from build123d import *

# Parameters (mm, degrees)
ESQUISSE1_R             = 4.25
BOSS_EXTRU_1_DEPTH      = 8
ESQUISSE2_W             = 5.5
ESQUISSE2_H             = 31
BOSS_EXTRU_2_DEPTH      = 1
CHANFREIN1_SIZE         = 1
ESQUISSE3_R             = 2.1
ENL_V_MAT_EXTRU_1_DEPTH = 39.288379438
ENL_V_START             = -5
ESQUISSE4_R             = 4
ENL_V_MAT_EXTRU_2_DEPTH = 33.749172176
CONG_1_R                = 2.5


with BuildPart() as part:
    # Esquisse1 → Boss.-Extru.1 (new, symmetric)
    with BuildSketch(Plane(origin=(0, 0, 0), x_dir=(0, 0, -1), z_dir=(1, 0, 0))):
        with BuildLine():
            Line((0, 0), (0, 31))
            Line((0, 31), (-10, 31))
            ThreePointArc((-10, 31), (-18.331958567, 26.529779962), (-19.214779507, 17.115693286))
            Line((-19.214779507, 17.115693286), (-12, 0))
            Line((-12, 0), (0, 0))
        make_face()
        with Locations((-10, 21)):
            Circle(ESQUISSE1_R, mode=Mode.SUBTRACT)
    extrude(amount=BOSS_EXTRU_1_DEPTH, both=True)

    # Esquisse2 → Boss.-Extru.2 (add)
    with BuildSketch(Plane(origin=(0, 0, 0), x_dir=(-1, 0, 0), z_dir=(0, 0, -1))):
        with Locations((0, 15.5)):
            Rectangle(ESQUISSE2_W, ESQUISSE2_H)
    extrude(amount=BOSS_EXTRU_2_DEPTH)

    # Chanfrein1
    chanfrein1_edges = [part.edges().sort_by_distance(p)[0] for p in [
        (-2.75, 15.5, -1),
        (2.75, 15.5, -1),
    ]]
    chamfer(chanfrein1_edges, length=CHANFREIN1_SIZE - 0.0001)  # a hair under: the kernel refuses the full size

    # Esquisse3 → Enlèv. mat.-Extru.1 (cut, through all)
    with BuildSketch(Plane(origin=(0, 0, -1), x_dir=(-1, 0, 0), z_dir=(0, 0, -1))):
        with Locations(Location((0, 10, 0), (0, 0, 326.442690238))):
            Circle(ESQUISSE3_R)
    extrude(amount=-ENL_V_MAT_EXTRU_1_DEPTH, mode=Mode.SUBTRACT)

    # Esquisse4 → Enlèv. mat.-Extru.2 (cut, through all)
    with BuildSketch(Plane(origin=(0, 0, 0), x_dir=(-1, 0, 0), z_dir=(0, 0, -1)).offset(ENL_V_START)):
        with Locations((0, 10)):
            Circle(ESQUISSE4_R)
    extrude(amount=-ENL_V_MAT_EXTRU_2_DEPTH, mode=Mode.SUBTRACT)

    # Congé1
    cong_1_edges = [part.edges().sort_by_distance(p)[0] for p in [
        (8, 31, 5),
        (8, 26.529779962, 18.331958567),
        (-8, 21, 14.25),
        (8, 21, 14.25),
        (8, 8.557846643, 15.607389753),
        (-8, 8.557846643, 15.607389753),
        (-8, 26.529779962, 18.331958567),
        (-8, 31, 5),
    ]]
    fillet(cong_1_edges, radius=CONG_1_R)


solid = part.part
Source: CAD feature listing. Evaluate the final solid. Frame: model axes, mm. A direction names the side the tool comes from. Coordinates: 2 decimals unless noted, no trailing zeros. Write each loop counter-clockwise with the first axis right and the second up, starting at its lowest first coordinate (ties: lowest second). Pieces come first, ordered by that corner, then holes. Notation, with made-up numbers: M 55,51.25 L 87,51.25 A13 ccw 87,68.25 Z; hole C 21,28 d7. An arc over 180 degrees is marked long. Use a Markdown table: item, result.
1) Mould query, pull axis Z, two halves, no side actions, for faces 1 (the cylindrical face through (0.521, 13.966, 9.942)), 2 (the flat face through (0, 4, -1)), 3 (the cylindrical face through (-0.08, 16.85, 10.92)), 4 (the cylindrical face through (7.287, 8.238, 14.657)). Classes: pulls with the +Z half, pulls with the -Z half, needs draft (parallel to the pull), parting line crosses it, or undercut.
Conclusion:
| item | result |
|---|---|
| face 1 | needs draft |
| face 2 | pulls with the -Z half |
| face 3 | undercut |
| face 4 | pulls with the +Z half |
2) Section A-A, the plane x = -0.5. Output: boundary loops of the cut face in (y, z).
Conclusion:
| item | result |
|---|---|
| outline | M 0,-1 L 7.96,-1 L 7.96,5 L 6.03,5 L 6.03,14.54 L 0,12 Z; M 12.04,-1 L 31,-1 L 31,10 A10 ccw 17.12,19.21 L 13.97,17.89 L 13.97,5 L 12.04,5 Z; hole C 21,10 d8.5 |
3) Reachability of faces 5 (the flat face through (-2, 8, 5)), 6 (the flat face through (-5, 15, 0)), 7 (the flat face through (5, 15, 0)), 8 (the flat face through (-8, 11, 5)), 9 (the flat face through (8, 11, 5)) from +Z, -Z, +X, -X, +Y, -Y: full face, straight path, thin tool, end or side. Return the list, or none.
Conclusion:
| item | result |
|---|---|
| face 5 | +Z |
| face 6 | -Z, -X, +Y, -Y |
| face 7 | -Z, +X, +Y, -Y |
| face 8 | +Z, -Z, -X, +Y, -Y |
| face 9 | +Z, -Z, +X, +Y, -Y |
4) First-contact query: pin 1 Ø7 at (y, z) = (21, 10) entering from +X; pin 2 Ø2.5 at (x, y) = (-5, 11.5) entering from -Z; pin 3 Ø6 at (x, z) = (2.5, 17.5) entering from -Y; pin 4 Ø1 at (x, z) = (-5.5, 13.5) entering from +Y. Flat tips, straight axial feed; report the tip coordinate or a pass-through.
Conclusion:
| item | result |
|---|---|
| pin 1 | passes through |
| pin 2 | stops at z = 0 |
| pin 3 | stops at y = 5.93 |
| pin 4 | stops at y = 30.54 |
5) Section B-B, the plane x = 4.75. Output: boundary loops of the cut face in (y, z), then the cut area to 3 significant figures.
Conclusion:
| item | result |
|---|---|
| outline | M 0,0 L 31,0 L 31,10 A10 ccw 17.12,19.21 L 0,12 Z; hole C 21,10 d8.5 |
| area | 466 mm^2 |
6) Ray query, L1, parallel to Y at x = -0.25, z = 10; L2, parallel to Y at x = 0, z = 1.75; L3, parallel to Z at x = -1, y = 12. Return the intervals inside material, ascending.
Conclusion:
| item | result |
|---|---|
| L1 | y = 0 to 6.01, 13.99 to 16.75, 25.25 to 31 |
| L2 | y = 0 to 7.9, 12.1 to 31 |
| L3 | z = -1 to 5 |
7) Section C-C, the plane z = 8.5. Give the number of separate pieces and of enclosed holes in the cut face, then the cut area to 3 significant figures.
Conclusion:
| item | result |
|---|---|
| separate pieces | 2 |
| enclosed holes | 1 |
| area | 310 mm^2 |
